Source: CAD feature listing. Evaluate the final solid. Frame: model axes, mm. A direction names the side the tool comes from. Give positions to 0.01 mm unless a question says otherwise; leave off trailing zeros. Order: outer loops, then holes, each group sorted by start corner. A loop starts at its lowest first (then second) coordinate and runs counter-clockwise, first axis right, second up. Notation, with made-up numbers: M -7,-23 L 22,-23 A29 cw 22,11 Z; hole C -39,-18.5 d7. An arc over 180 degrees is marked long. Answer as a JSON object with one key per item and string values. Group by question number.
1. Set-up query: faces 1 (the flat face through (0, -25, 1)), 2 (the cylindrical face through (53.214, -12.456, 1.521)). Return all of +Z, -Z, +X, -X, +Y, -Y with unobstructed straight access to the full face (end or side cutting, diameter ignored); none if empty.
2. Pull-direction query (X, two-part tool) for faces 3 (the flat face through (82, -29, 3)), 4 (the cylindrical face through (38.82, -27.58, 1.52)), 5 (the cylindrical face through (1, -43, 2)), 6 (the cylindrical face through (57.079, -8.063, 1.521)); classes: +X half, -X half, draft (parallel to the pull), parting line (faces both ways), or undercut.
3. Section query B-B (y = -24). Output: boundary loops of the cut face in (x, z).
4. Material intervals for L1, parallel to Y at x = 104.5, z = 1.45; L2, parallel to Y at x = 119, z = 0.6; L3, parallel to X at y = -32, z = 2.1, sorted ascending. Write a range as [from, to].
5. Section query C-C (z = 1.6). Count the separate pieces of the cut face and the enclosed holes in it, plus the area to 3 significant figures.
6. Section query A-A (x = 69.5). Output: boundary loops of the cut face in (y, z), plus the area to 3 significant figures.
from build123d import *

# Parameters (mm, degrees)
SKETCH_1_W          = 174
SKETCH_1_H          = 45
SKETCH_1_R          = 2
EXTRUDE_1_DEPTH     = 3
SKETCH_2_R          = 1.25
CUT_EXTRUDE_1_DEPTH = 3
SKETCH_3_W          = 20
SKETCH_3_H          = 10
CUT_EXTRUDE_2_DEPTH = 4
FILLET_1_R          = 2
FILLET_2_R          = 5
SKETCH_4_W          = 93.235772227
SKETCH_4_H          = 5
CUT_EXTRUDE_3_DEPTH = 4
FILLET_3_R          = 5


with BuildPart() as part:
    # 草图1 → 凸台-拉伸1 (new body)
    with BuildSketch(Plane.XY):
        with Locations((87, -22.5)):
            Rectangle(SKETCH_1_W, SKETCH_1_H)
        with Locations((69.5, -10.5)):
            Circle(SKETCH_1_R, mode=Mode.SUBTRACT)
        with Locations(Location((104.5, -10.5, 0), (0, 0, 180))):
            Circle(SKETCH_1_R, mode=Mode.SUBTRACT)
        with Locations(Location((69.5, -34.5, 0), (0, 0, 180))):
            Circle(SKETCH_1_R, mode=Mode.SUBTRACT)
        with Locations((104.5, -34.5)):
            Circle(SKETCH_1_R, mode=Mode.SUBTRACT)
    extrude(amount=EXTRUDE_1_DEPTH)

    # 草图2 → 切除-拉伸1 (cut)
    with BuildSketch(Plane.XY.offset(3)):
        with Locations((148, -20)):
            Circle(SKETCH_2_R)
        with Locations((148, -40)):
            Circle(SKETCH_2_R)
        with Locations(Location((26, -40, 0), (0, 0, 180))):
            Circle(SKETCH_2_R)
        with Locations(Location((26, -20, 0), (0, 0, 180))):
            Circle(SKETCH_2_R)
        with Locations((4, -20)):
            Circle(SKETCH_2_R)
        with Locations((4, -40)):
            Circle(SKETCH_2_R)
        with Locations(Location((170, -40, 0), (0, 0, 180))):
            Circle(SKETCH_2_R)
        with Locations(Location((170, -20, 0), (0, 0, 180))):
            Circle(SKETCH_2_R)
    extrude(amount=-CUT_EXTRUDE_1_DEPTH, mode=Mode.SUBTRACT)

    # 草图3 → 切除-拉伸2 (cut)
    with BuildSketch(Plane.XY.offset(3)):
        Polygon((6.964585687, -8.446455347), (15.15178831, -8.446455347), (6.964585687, -12.03733369), align=None)
        Polygon((6.964585687, -14.220208877), (23.031657012, -7.17324777), (23.031657012, -14.220208877), align=None)
        Polygon((37.415694542, -6.798433242), (47.456920401, -18.258527972), (37.415694542, -31.683210371), align=None)
        Polygon((47.456920401, -6.798433242), (53.137279326, -13.281451581), (60.536376343, -6.798433242), align=None)
        Polygon((47.456920401, -34.411804354), (61.610874696, -15.488582851), (61.610874696, -40.632998636), align=None)
        Polygon((112.389125304, -40.632998636), (126.543079599, -34.411804354), (112.389125304, -15.488582851), align=None)
        Polygon((113.463623657, -6.798433242), (126.543079599, -6.798433242), (120.862720674, -13.281451581), align=None)
        Polygon((136.584305458, -31.683210371), (136.584305458, -6.798433242), (126.543079599, -18.258527972), align=None)
        Polygon((150.968342988, -14.220208877), (167.035414313, -14.220208877), (150.968342988, -7.17324777), align=None)
        Polygon((167.035414313, -12.03733369), (167.035414313, -8.446455347), (158.84821169, -8.446455347), align=None)
        with Locations((87, -22.950058647)):
            Rectangle(SKETCH_3_W, SKETCH_3_H)
    extrude(amount=-CUT_EXTRUDE_2_DEPTH, mode=Mode.SUBTRACT)

    # 圆角1
    # the kernel refuses this fillet: 2 mm, written as the material it adds along each edge
    with BuildSketch(Plane(origin=(15.15178831, -8.446455347, 3), x_dir=(-0.9157882087939493, -0.40166149508506527, 0), z_dir=(0, 0, -1)), Plane(origin=(167.035414313, -14.220208877, 3), x_dir=(-1, 0, 0), z_dir=(0, 0, -1))) as fillet_1_piece_1:
        with BuildLine():
            CenterArc((FILLET_1_R * 4.76965861114, FILLET_1_R), FILLET_1_R, 113.682087725, 156.317912275)
            Line((FILLET_1_R * 4.36799711605, FILLET_1_R * 1.91578820879), (0, 0))
            Line((0, 0), (FILLET_1_R * 4.76965861114, 0))
        make_face()
    extrude(amount=3)
    with BuildSketch(Plane(origin=(6.964585687, -12.03733369, 3), x_dir=(0.9157882087939492, 0.4016614950850657, 0), z_dir=(0, 0, -1)), Plane(origin=(167.035414313, -12.03733369, 3), x_dir=(0, 1, 0), z_dir=(0, 0, -1)), Plane(origin=(150.968342988, -7.17324777, 3), x_dir=(0, -1, 0), z_dir=(0, 0, -1))) as fillet_1_piece_2:
        with BuildLine():
            CenterArc((FILLET_1_R * 1.53055202243, -FILLET_1_R), FILLET_1_R, 90, 113.682087725)
            Line((FILLET_1_R * 0.614763813634, -FILLET_1_R * 1.40166149509), (0, 0))
            Line((0, 0), (FILLET_1_R * 1.53055202243, 0))
        make_face()
    extrude(amount=3)
    with BuildSketch(Plane(origin=(6.964585687, -8.446455347, 3), x_dir=(0, -1, 0), z_dir=(0, 0, -1)), Plane(origin=(77, -27.950058647, 3), x_dir=(1, 0, 0), z_dir=(0, 0, -1)), Plane(origin=(77, -17.950058647, 3), x_dir=(0, -1, 0), z_dir=(0, 0, -1)), Plane(origin=(97, -17.950058647, 3), x_dir=(-1, 0, 0), z_dir=(0, 0, -1)), Plane(origin=(120.862720674, -13.281451581, 3), x_dir=(0.6590115853993712, 0.752132787684068, 0), z_dir=(0, 0, -1)), Plane(origin=(150.968342988, -14.220208877, 3), x_dir=(1, 0, 0), z_dir=(0, 0, -1)), Plane(origin=(23.031657012, -14.220208877, 3), x_dir=(0, 1, 0), z_dir=(0, 0, -1))) as fillet_1_piece_3:
        with BuildLine():
            CenterArc((FILLET_1_R, -FILLET_1_R), FILLET_1_R, 90, 90)
            Line((0, -FILLET_1_R), (0, 0))
            Line((0, 0), (FILLET_1_R, 0))
        make_face()
    extrude(amount=3)
    with BuildSketch(Plane(origin=(97, -27.950058647, 3), x_dir=(-1, 0, 0), z_dir=(0, 0, -1)), Plane(origin=(167.035414313, -8.446455347, 3), x_dir=(0, -1, 0), z_dir=(0, 0, -1)), Plane(origin=(53.137279326, -13.281451581, 3), x_dir=(-0.6590115853993732, 0.7521327876840662, 0), z_dir=(0, 0, -1))) as fillet_1_piece_4:
        with BuildLine():
            CenterArc((FILLET_1_R, FILLET_1_R), FILLET_1_R, 180, 90)
            Line((0, FILLET_1_R), (0, 0))
            Line((0, 0), (FILLET_1_R, 0))
        make_face()
    extrude(amount=3)
    with BuildSketch(Plane(origin=(158.84821169, -8.446455347, 3), x_dir=(0.9157882087939491, -0.40166149508506555, 0), z_dir=(0, 0, -1)), Plane(origin=(6.964585687, -14.220208877, 3), x_dir=(1, 0, 0), z_dir=(0, 0, -1))) as fillet_1_piece_5:
        with BuildLine():
            CenterArc((FILLET_1_R * 4.76965861114, -FILLET_1_R), FILLET_1_R, 90, 156.317912275)
            Line((FILLET_1_R * 4.36799711605, -FILLET_1_R * 1.91578820879), (0, 0))
            Line((0, 0), (FILLET_1_R * 4.76965861114, 0))
        make_face()
    extrude(amount=3)
    with BuildSketch(Plane(origin=(126.543079599, -34.411804354, 3), x_dir=(-0.9154710305438037, -0.40238388664938624, 0), z_dir=(0, 0, -1))) as fillet_1_piece_6:
        with BuildLine():
            CenterArc((FILLET_1_R * 1.25870478162, FILLET_1_R), FILLET_1_R, 166.931997768, 103.068002232)
            Line((FILLET_1_R * 0.284602389093, FILLET_1_R * 1.22610733927), (0, 0))
            Line((0, 0), (FILLET_1_R * 1.25870478162, 0))
        make_face()
    extrude(amount=3)
    with BuildSketch(Plane(origin=(112.389125304, -40.632998636, 3), x_dir=(0.9154710305438044, 0.4023838866493844, 0), z_dir=(0, 0, -1)), Plane(origin=(61.610874696, -40.632998636, 3), x_dir=(0, 1, 0), z_dir=(0, 0, -1))) as fillet_1_piece_7:
        with BuildLine():
            CenterArc((FILLET_1_R * 1.53187139719, -FILLET_1_R), FILLET_1_R, 90, 113.727291576)
            Line((FILLET_1_R * 0.61640036665, -FILLET_1_R * 1.40238388665), (0, 0))
            Line((0, 0), (FILLET_1_R * 1.53187139719, 0))
        make_face()
    extrude(amount=3)
    with BuildSketch(Plane(origin=(112.389125304, -15.488582851, 3), x_dir=(0, -1, 0), z_dir=(0, 0, -1)), Plane(origin=(136.584305458, -31.683210371, 3), x_dir=(0, 1, 0), z_dir=(0, 0, -1)), Plane(origin=(37.415694542, -31.683210371, 3), x_dir=(0.5989578255907083, 0.8007805711701868, 0), z_dir=(0, 0, -1))) as fillet_1_piece_8:
        with BuildLine():
            CenterArc((FILLET_1_R * 3.00652315444, -FILLET_1_R), FILLET_1_R, 90, 143.204706192)
            Line((FILLET_1_R * 2.40756532885, -FILLET_1_R * 1.80078057117), (0, 0))
            Line((0, 0), (FILLET_1_R * 3.00652315444, 0))
        make_face()
    extrude(amount=3)
    with BuildSketch(Plane(origin=(126.543079599, -6.798433242, 3), x_dir=(-0.6590115853993721, -0.7521327876840671, 0), z_dir=(0, 0, -1))) as fillet_1_piece_9:
        with BuildLine():
            CenterArc((FILLET_1_R * 2.2057429387, FILLET_1_R), FILLET_1_R, 138.775465824, 131.224534176)
            Line((FILLET_1_R * 1.45361015102, FILLET_1_R * 1.6590115854), (0, 0))
            Line((0, 0), (FILLET_1_R * 2.2057429387, 0))
        make_face()
    extrude(amount=3)
    with BuildSketch(Plane(origin=(113.463623657, -6.798433242, 3), x_dir=(0.752132787684067, -0.6590115853993724, 0), z_dir=(0, 0, -1)), Plane(origin=(37.415694542, -6.798433242, 3), x_dir=(0, -1, 0), z_dir=(0, 0, -1)), Plane(origin=(60.536376343, -6.798433242, 3), x_dir=(-1, 0, 0), z_dir=(0, 0, -1))) as fillet_1_piece_10:
        with BuildLine():
            CenterArc((FILLET_1_R * 2.65872835395, -FILLET_1_R), FILLET_1_R, 90, 138.775465824)
            Line((FILLET_1_R * 1.99971676855, -FILLET_1_R * 1.75213278768), (0, 0))
            Line((0, 0), (FILLET_1_R * 2.65872835395, 0))
        make_face()
    extrude(amount=3)
    with BuildSketch(Plane(origin=(136.584305458, -6.798433242, 3), x_dir=(0, -1, 0), z_dir=(0, 0, -1))) as fillet_1_piece_11:
        with BuildLine():
            CenterArc((FILLET_1_R * 2.65872835395, FILLET_1_R), FILLET_1_R, 131.224534176, 138.775465824)
            Line((FILLET_1_R * 1.99971676855, FILLET_1_R * 1.75213278768), (0, 0))
            Line((0, 0), (FILLET_1_R * 2.65872835395, 0))
        make_face()
    extrude(amount=3)
    with BuildSketch(Plane(origin=(23.031657012, -7.17324777, 3), x_dir=(0, -1, 0), z_dir=(0, 0, -1))) as fillet_1_piece_12:
        with BuildLine():
            CenterArc((FILLET_1_R * 1.53055202243, FILLET_1_R), FILLET_1_R, 156.317912275, 113.682087725)
            Line((FILLET_1_R * 0.614763813634, FILLET_1_R * 1.40166149509), (0, 0))
            Line((0, 0), (FILLET_1_R * 1.53055202243, 0))
        make_face()
    extrude(amount=3)
    with BuildSketch(Plane(origin=(47.456920401, -18.258527972, 3), x_dir=(-0.5989578255907079, -0.8007805711701871, 0), z_dir=(0, 0, -1))) as fillet_1_piece_13:
        with BuildLine():
            CenterArc((FILLET_1_R * 0.810070570787, FILLET_1_R), FILLET_1_R, 191.980172016, 78.019827984)
            Line((-FILLET_1_R * 0.168148922043, FILLET_1_R * 0.792426822912), (0, 0))
            Line((0, 0), (FILLET_1_R * 0.810070570787, 0))
        make_face()
    extrude(amount=3)
    with BuildSketch(Plane(origin=(47.456920401, -6.798433242, 3), x_dir=(0.6590115853993722, -0.752132787684067, 0), z_dir=(0, 0, -1))) as fillet_1_piece_14:
        with BuildLine():
            CenterArc((FILLET_1_R * 2.2057429387, -FILLET_1_R), FILLET_1_R, 90, 131.224534176)
            Line((FILLET_1_R * 1.45361015102, -FILLET_1_R * 1.6590115854), (0, 0))
            Line((0, 0), (FILLET_1_R * 2.2057429387, 0))
        make_face()
    extrude(amount=3)
    with BuildSketch(Plane(origin=(61.610874696, -15.488582851, 3), x_dir=(0, -1, 0), z_dir=(0, 0, -1))) as fillet_1_piece_15:
        with BuildLine():
            CenterArc((FILLET_1_R * 3.00652315444, FILLET_1_R), FILLET_1_R, 126.795293808, 143.204706192)
            Line((FILLET_1_R * 2.40756532885, FILLET_1_R * 1.80078057117), (0, 0))
            Line((0, 0), (FILLET_1_R * 3.00652315444, 0))
        make_face()
    extrude(amount=3)
    with BuildSketch(Plane(origin=(47.456920401, -34.411804354, 3), x_dir=(0.9154710305438037, -0.40238388664938624, 0), z_dir=(0, 0, -1))) as fillet_1_piece_16:
        with BuildLine():
            CenterArc((FILLET_1_R * 1.25870478162, -FILLET_1_R), FILLET_1_R, 90, 103.068002232)
            Line((FILLET_1_R * 0.284602389093, -FILLET_1_R * 1.22610733927), (0, 0))
            Line((0, 0), (FILLET_1_R * 1.25870478162, 0))
        make_face()
    extrude(amount=3)
    with BuildSketch(Plane(origin=(126.543079599, -18.258527972, 3), x_dir=(0.5989578255907072, -0.8007805711701876, 0), z_dir=(0, 0, -1))) as fillet_1_piece_17:
        with BuildLine():
            CenterArc((FILLET_1_R * 0.810070570787, -FILLET_1_R), FILLET_1_R, 90, 78.019827984)
            Line((-FILLET_1_R * 0.168148922043, -FILLET_1_R * 0.792426822912), (0, 0))
            Line((0, 0), (FILLET_1_R * 0.810070570787, 0))
        make_face()
    extrude(amount=3)

    # 圆角2
    fillet_2_edges = [part.edges().sort_by_distance(p)[0] for p in [
        (0, 0, 1.5),
        (174, 0, 1.5),
        (174, -45, 1.5),
        (0, -45, 1.5),
    ]]
    fillet(fillet_2_edges, radius=FILLET_2_R)

    # 草图4 → 切除-拉伸3 (cut)
    with BuildSketch(Plane.XY.offset(3)):
        with Locations((127.382113887, -2.5)):
            Rectangle(SKETCH_4_W, SKETCH_4_H)
        with Locations((46.617886114, -2.5)):
            Rectangle(SKETCH_4_W, SKETCH_4_H)
    extrude(amount=-CUT_EXTRUDE_3_DEPTH, mode=Mode.SUBTRACT)

    # 圆角3
    fillet_3_edges = [part.edges().sort_by_distance(p)[0] for p in [
        (0, -5, 1.5),
        (174, -5, 1.5),
    ]]
    fillet(fillet_3_edges, radius=FILLET_3_R)


solid = part.part
Answer sheet:
{
 "1": {"face 1": "+Z, -Z, -X, +Y, -Y", "face 2": "+Z, -Z"},
 "2": {"face 3": "draft", "face 4": "undercut", "face 5": "-X half", "face 6": "undercut"},
 "3": {"outline": "M 0,0 L 37.42,0 L 37.42,3 L 0,3 Z; M 43.16,0 L 55.24,0 L 55.24,3 L 43.16,3 Z; M 61.61,0 L 77,0 L 77,3 L 61.61,3 Z; M 97,0 L 112.39,0 L 112.39,3 L 97,3 Z; M 118.76,0 L 130.84,0 L 130.84,3 L 118.76,3 Z; M 136.58,0 L 174,0 L 174,3 L 136.58,3 Z"},
 "4": {"L1": "[-45, -36.5], [-32.5, -12.5], [-8.5, -5]", "L2": "[-45, -37.73], [-24.33, -11.65], [-6.8, -5]", "L3": "[0, 49.26], [61.61, 112.39], [124.74, 174]"},
 "5": {"separate pieces": "1", "enclosed holes": "23", "area": "5,950 mm^2"},
 "6": {"outline": "M -45,0 L -36.5,0 L -36.5,3 L -45,3 Z; M -32.5,0 L -12.5,0 L -12.5,3 L -32.5,3 Z; M -8.5,0 L -5,0 L -5,3 L -8.5,3 Z", "area": "96.0 mm^2"}
}
